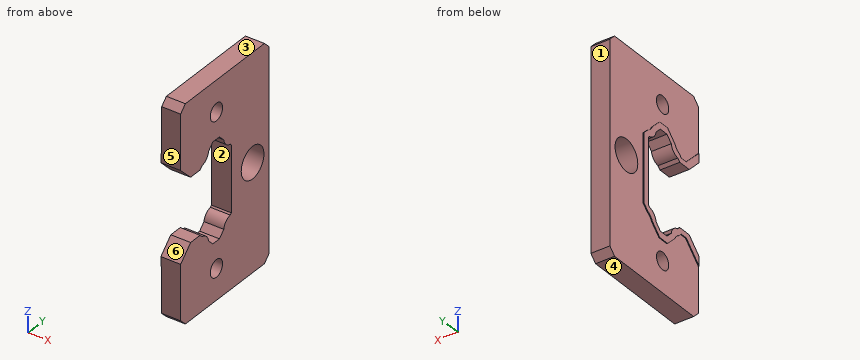
```python
from build123d import *

# Parameters (mm, degrees)
EXTRUDE_1_DEPTH          = 1.5
EXTRUDE_1_DEPTH_BACK     = 1.5
CUT_EXTRUDE_1_DEPTH      = 1.5
CUT_EXTRUDE_1_DEPTH_BACK = 1.5
CUT_EXTRUDE_2_DEPTH      = 0.12
SKETCH_4_R               = 2.4
CUT_EXTRUDE_3_DEPTH      = 3
CUT_EXTRUDE_4_DEPTH      = 3
CUT_EXTRUDE_4_DEPTH_BACK = 3
SKETCH_5_R               = 1.3
CUT_EXTRUDE_5_DEPTH      = 3
CUT_EXTRUDE_5_DEPTH_BACK = 3
SKETCH_6_R               = 1.3


with BuildPart() as part:
    # Эскиз1 → Бобышка-Вытянуть1 (new, two sides: drawn at the far end of the back side and taken through both)
    with BuildSketch(Plane(origin=(0, 0, 0), x_dir=(0, 0, -1), z_dir=(1, 0, 0)).offset(-EXTRUDE_1_DEPTH_BACK)):
        Polygon((-16.2, 0.997020561), (-15.202979439, 0), (15.202979439, 0), (16.2, 0.997020561), (16.2, 17.702979439), (15.202979439, 18.7), (-15.202979439, 18.7), (-16.2, 17.702979439), align=None)
    extrude(amount=EXTRUDE_1_DEPTH + EXTRUDE_1_DEPTH_BACK)

    # Эскиз2 → Вырез-Вытянуть1 (cut, two sides: drawn at the far end of the back side and taken through both)
    with BuildSketch(Plane(origin=(0, 0, 0), x_dir=(0, 0, -1), z_dir=(1, 0, 0)).offset(-CUT_EXTRUDE_1_DEPTH_BACK)):
        with BuildLine():
            Line((-11.2, -4.3), (11.2, -4.3))
            Line((11.2, -4.3), (4.8, 2.1))
            Line((4.8, 2.1), (4.8, 4.1))
            Line((4.8, 4.1), (5.21443454, 4.51443454))
            ThreePointArc((5.21443454, 4.51443454), (5.66862915, 5.43137085), (6.58556546, 5.88556546))
            Line((6.58556546, 5.88556546), (7.5, 6.8))
            Line((7.5, 6.8), (7.5, 8.2))
            Line((7.5, 8.2), (6.58556546, 9.11443454))
            ThreePointArc((6.58556546, 9.11443454), (5.66862915, 9.56862915), (5.21443454, 10.48556546))
            Line((5.21443454, 10.48556546), (5, 10.7))
            Line((5, 10.7), (-5, 10.7))
            Line((-5, 10.7), (-5.21443454, 10.48556546))
            ThreePointArc((-5.21443454, 10.48556546), (-5.66862915, 9.56862915), (-6.58556546, 9.11443454))
            Line((-6.58556546, 9.11443454), (-7.5, 8.2))
            Line((-7.5, 8.2), (-7.5, 6.8))
            Line((-7.5, 6.8), (-6.58556546, 5.88556546))
            ThreePointArc((-6.58556546, 5.88556546), (-5.66862915, 5.43137085), (-5.21443454, 4.51443454))
            Line((-5.21443454, 4.51443454), (-4.8, 4.1))
            Line((-4.8, 4.1), (-4.8, 2.1))
            Line((-4.8, 2.1), (-11.2, -4.3))
        make_face()
    extrude(amount=CUT_EXTRUDE_1_DEPTH + CUT_EXTRUDE_1_DEPTH_BACK, mode=Mode.SUBTRACT)

    # Эскиз3 → Вырез-Вытянуть2 (cut)
    with BuildSketch(Plane(origin=(-1.5, 0, 0), x_dir=(0, 0, -1), z_dir=(1, 0, 0))):
        with BuildLine():
            Line((-16.2, -4.3), (-12.614213562, -4.3))
            Line((-12.614213562, -4.3), (-5.6, 2.714213562))
            Line((-5.6, 2.714213562), (-5.6, 3.76862915))
            Line((-5.6, 3.76862915), (-6.023597697, 4.192226848))
            ThreePointArc((-6.023597697, 4.192226848), (-6.375735931, 4.724264069), (-6.907773152, 5.076402303))
            Line((-6.907773152, 5.076402303), (-8.5, 6.66862915))
            Line((-8.5, 6.66862915), (-8.5, 8.33137085))
            Line((-8.5, 8.33137085), (-6.907773152, 9.923597697))
            ThreePointArc((-6.907773152, 9.923597697), (-6.375735931, 10.275735931), (-6.023597697, 10.807773152))
            Line((-6.023597697, 10.807773152), (-5.13137085, 11.7))
            Line((-5.13137085, 11.7), (5.13137085, 11.7))
            Line((5.13137085, 11.7), (6.023597697, 10.807773152))
            ThreePointArc((6.023597697, 10.807773152), (6.375735931, 10.275735931), (6.907773152, 9.923597697))
            Line((6.907773152, 9.923597697), (8.5, 8.33137085))
            Line((8.5, 8.33137085), (8.5, 6.66862915))
            Line((8.5, 6.66862915), (6.907773152, 5.076402303))
            ThreePointArc((6.907773152, 5.076402303), (6.375735931, 4.724264069), (6.023597697, 4.192226848))
            Line((6.023597697, 4.192226848), (5.6, 3.76862915))
            Line((5.6, 3.76862915), (5.6, 2.714213562))
            Line((5.6, 2.714213562), (12.614213562, -4.3))
            Line((12.614213562, -4.3), (16.2, -4.3))
            Line((16.2, -4.3), (16.2, 18.7))
            Line((16.2, 18.7), (-16.2, 18.7))
            Line((-16.2, 18.7), (-16.2, -4.3))
        make_face()
    extrude(amount=CUT_EXTRUDE_2_DEPTH, mode=Mode.SUBTRACT)

    # Эскиз4 → Вырез-Вытянуть3 (cut)
    with BuildSketch(Plane(origin=(-1.5, 0, 0), x_dir=(0, 0, -1), z_dir=(1, 0, 0))):
        with Locations((0, 15.2)):
            Circle(SKETCH_4_R)
    extrude(amount=CUT_EXTRUDE_3_DEPTH, mode=Mode.SUBTRACT)

    # Эскиз5 → Вырез-Вытянуть4 (cut, two sides: drawn at the far end of the back side and taken through both)
    with BuildSketch(Plane(origin=(0, 0, 0), x_dir=(0, 0, -1), z_dir=(1, 0, 0)).offset(-CUT_EXTRUDE_4_DEPTH_BACK)):
        with Locations((-11.5, 7.555556)):
            Circle(SKETCH_5_R)
    extrude(amount=CUT_EXTRUDE_4_DEPTH + CUT_EXTRUDE_4_DEPTH_BACK, mode=Mode.SUBTRACT)

    # Эскиз6 → Вырез-Вытянуть5 (cut, two sides: drawn at the far end of the back side and taken through both)
    with BuildSketch(Plane(origin=(0, 0, 0), x_dir=(0, 0, -1), z_dir=(1, 0, 0)).offset(-CUT_EXTRUDE_5_DEPTH_BACK)):
        with Locations((11.5, 7.555556)):
            Circle(SKETCH_6_R)
    extrude(amount=CUT_EXTRUDE_5_DEPTH + CUT_EXTRUDE_5_DEPTH_BACK, mode=Mode.SUBTRACT)


solid = part.part
```
Verification items for the finished model (mm, model axes). Face numbers are marked on the shaded views. A direction names the side the tool comes from. Coordinates: 2 decimals unless noted, no trailing zeros. Write each loop counter-clockwise with the first axis right and the second up, starting at its lowest first coordinate (ties: lowest second). Pieces come first, ordered by that corner, then holes. Notation, with made-up numbers: M -37,26.25 L -5,26.25 A19 ccw -5,60.25 Z; hole C 12.5,-5 d7. An arc over 180 degrees is marked long. Answer as a JSON object with one key per item and string values. Group by question number.
(1) Material ranges on line 1 (Y direction, x = 0.45, z = -11.5); line 2 (Y direction, x = -0.5, z = 0); line 3 (Z direction, x = -0.6, y = 15.2), recorded low to high.
(2) Tool access check on the marked faces 5 and 6. Record the directions out of +Z, -Z, +X, -X, +Y, -Y that give a thin tool (end or side, any length) a straight path to the whole face; none if there is none.
(3) Cross-section at B-B, the plane z = 0. Record the cut outline in (x, y).
(4) Cross-section at D-D, the plane z = -11.5. Record the cut outline in (x, y).
(5) Cross-section at A-A, the plane y = 15.2. Record the cut outline in (x, z), and give its area (3 significant figures).
(6) Gauge pin test, flat ends, axial feed: pin 1 (5 mm diameter, centred on y = 3.5, z = 1.5, fed in from -X); pin 2 (1.5 mm diameter, centred on x = 1, z = -3.5, fed in from -Y); pin 3 (1 mm diameter, centred on x = 1, z = 4.5, fed in from -Y); pin 4 (4 mm diameter, centred on y = 7.56, z = 11.5, fed in from -X). Record the tip position at first contact, or that the pin passes through.
(7) Release check for a two-part mould opening along Z. For the marked faces 1, 2, 3 and 4 record: +Z half, -Z half, draft (parallel to the pull), parting line (faces both ways), or undercut.
(8) Cross-section at C-C, the plane x = -0.8. State how many separate pieces and enclosed holes the cut face has, and give its area (3 significant figures).
Reply:
{
 "1": {"line 1": "0 to 6.26, 8.86 to 18.7", "line 2": "10.7 to 12.8, 17.6 to 18.7", "line 3": "-16.2 to -2.4, 2.4 to 16.2"},
 "2": {"face 5": "+Z, -Z, +X, -X, -Y", "face 6": "+X, -X, -Y"},
 "3": {"outline": "M -1.5,10.7 L 1.5,10.7 L 1.5,12.8 L -1.38,12.8 L -1.38,11.7 L -1.5,11.7 Z; M -1.38,17.6 L 1.5,17.6 L 1.5,18.7 L -1.38,18.7 Z"},
 "4": {"outline": "M -1.38,0 L 1.5,0 L 1.5,6.26 L -1.38,6.26 Z; M -1.38,8.86 L 1.5,8.86 L 1.5,18.7 L -1.38,18.7 Z"},
 "5": {"outline": "M -1.38,-16.2 L 1.5,-16.2 L 1.5,-2.4 L -1.38,-2.4 Z; M -1.38,2.4 L 1.5,2.4 L 1.5,16.2 L -1.38,16.2 Z", "area": "79.5 mm²"},
 "6": {"pin 1": "through", "pin 2": "y = 10.7", "pin 3": "y = 1.9", "pin 4": "x = -1.38"},
 "7": {"face 1": "draft", "face 2": "undercut", "face 3": "+Z half", "face 4": "-Z half"},
 "8": {"separate pieces": "1", "enclosed holes": "3", "area": "448 mm²"}
}
